from build123d import *

# Parameters (mm, degrees)
F0_W     = 112
F0_H     = 13.5
F2_DEPTH = 117.5
F3_DEPTH = 15
F4_R     = 6
F5_DEPTH = 20
F6_DEPTH = 70


with BuildPart() as f1:
    # F0 (on Front) → F1 (revolve)
    with BuildSketch(Plane.XZ):
        with BuildLine():
            Line((84.7845596923, 37.8570006367), (84.7845596923, 55.8570006367))
            Line((84.7845596923, 55.8570006367), (84.7845596923, 61.6070006367))
            Line((84.7845596923, 61.6070006367), (68.7845596923, 61.6070006367))
            ThreePointArc((68.7845596923, 61.6070006367), (66.0366424473, 58.8617238614), (62.2845596923, 57.8570006367))
            Line((62.2845596923, 57.8570006367), (-42.2154403077, 57.8570006367))
            Line((-42.2154403077, 57.8570006367), (-42.2154403077, 55.8570006367))
            Line((-42.2154403077, 55.8570006367), (-52.2154403077, 55.8570006367))
            Line((-52.2154403077, 55.8570006367), (-52.2154403077, 56.2570006367))
            Line((-52.2154403077, 56.2570006367), (-55.2154403077, 56.2570006367))
            Line((-55.2154403077, 56.2570006367), (-55.2154403077, 51.3570006367))
            Line((-55.2154403077, 51.3570006367), (-43.2154403077, 51.3570006367))
            Line((-43.2154403077, 51.3570006367), (68.7845596923, 51.3570006367))
            Line((68.7845596923, 51.3570006367), (68.7845596923, 37.8570006367))
            Line((68.7845596923, 37.8570006367), (84.7845596923, 37.8570006367))
        make_face()
        with Locations((12.7845596923, 44.6070006367)):
            Rectangle(F0_W, F0_H)
    revolve(axis=Axis((14.7845596923, 0, 37.8570006367), (1, 0, 0)))

    # F2 (cut): a face of the model
    f2_faces = [f1.faces().sort_by_distance(p)[0] for p in [
        (-43.2154403077, 0, 37.8570006367),
    ]]
    extrude(f2_faces, amount=-F2_DEPTH, mode=Mode.SUBTRACT)

    # F0 (on Front) → F3 (join, symmetric)
    with BuildSketch(Plane.XZ):
        with BuildLine():
            Line((84.7845596923, 28.8570006367), (109.7845596923, 28.8570006367))
            ThreePointArc((109.7845596923, 28.8570006367), (100.8051004109, 37.2492909907), (108.5719143545, 46.7749315225))
            ThreePointArc((108.5719143545, 46.7749315225), (96.2900045696, 50.299124768), (84.7845596923, 55.8570006367))
            Line((84.7845596923, 55.8570006367), (84.7845596923, 37.8570006367))
            Line((84.7845596923, 37.8570006367), (84.7845596923, 28.8570006367))
        make_face()
        with BuildLine():
            ThreePointArc((108.5719143545, 46.7749315225), (100.8051004109, 37.2492909907), (109.7845596923, 28.8570006367))
            ThreePointArc((109.7845596923, 28.8570006367), (116.148520723, 31.493039606), (118.7845596923, 37.8570006367))
            ThreePointArc((118.7845596923, 37.8570006367), (115.70428063, 44.6361527975), (108.5719143545, 46.7749315225))
        make_face()
    extrude(amount=F3_DEPTH, both=True)

    # F4 (on face) → F5 (join)
    with BuildSketch(Plane.XZ.offset(15)):
        with Locations((109.7845596923, 37.8570006367)):
            Circle(F4_R)
    extrude(amount=F5_DEPTH)

    # F6 (add): a face of the model
    f6_faces = [f1.faces().sort_by_distance(p)[0] for p in [
        (109.7845596923, -35, 37.8570006367),
    ]]
    extrude(f6_faces, amount=-F6_DEPTH)


solid = f1.part
Read the model definition and answer for the solid it produces. Units are mm, in the model's axes. A direction names the side the tool comes from. Round coordinates to 2 decimals unless told otherwise and drop trailing zeros. Order: outer loops, then holes, each group sorted by start corner. A loop starts at its lowest first (then second) coordinate and runs counter-clockwise, first axis right, second up.
1) The mould has two halves that part along X. Classify faces 5 (the face through (103.79, 24.86, 38.12)), 6 (the face through (-55.215, -10, 28)), 7 (the face through (-53.736, -0.809, 19.475)): released by +X, released by -X, zero draft, split by the parting line, or undercut.
2) The part is cut by section A-A on y = 0. Write down the section's boundary in (x, z), plus the area to 3 significant figures.
3) The part is cut by section C-C on y = 27.5. Write down the section's boundary in (x, z).
4) Straight lines are drawn through the part: L1, parallel to Z at x = 33, y = 0; L2, parallel to Z at x = -48.75, y = 0; L3, parallel to Y at x = -38, z = 33.5. For each, find the intervals that lie inside material, in ascending order.
5) Flat-ended cylindrical pins translate along their axes: pin 1 (1.5 mm diameter, centred on x = -33.5, z = 22, fed in from -Y); pin 2 (4 mm diameter, centred on x = 4, y = 15, fed in from +Z); pin 3 (3 mm diameter, centred on x = 61.5, z = 53, fed in from +Y). Find the tip coordinate at first contact, or state that the pin passes through.
6) The part is cut by section B-B on x = -7. Write down the section's boundary in (y, z), plus the area to 3 significant figures.
7) For faces 1 (the face through (103.79, -24.86, 38.12)), 2 (the face through (97, 0, 28.857)), 3 (the face through (-42.215, -8, 21)), 4 (the face through (74.285, 0, 38)), determine the directions among +Z, -Z, +X, -X, +Y, -Y from which every point of the face is accessible in a straight line to the end or side of a thin tool.
Resolved:
1. face 5: undercut
1. face 6: released by -X
1. face 7: zero draft
2. outline: (-55.22, 19.46) - (-52.22, 19.46) - (-52.22, 19.86) - (-42.22, 19.86) - (-42.22, 17.86) - (62.28, 17.86) arc R7.51 cw to (68.78, 14.11) - (84.78, 14.11) - (84.78, 28.86) - (109.78, 28.86) arc R9 ccw (long way) to (108.57, 46.77) arc R75 cw to (84.78, 55.86) - (84.78, 61.61) - (68.78, 61.61) arc R7.51 cw to (62.28, 57.86) - (-42.22, 57.86) - (-42.22, 55.86) - (-52.22, 55.86) - (-52.22, 56.26) - (-55.22, 56.26) - (-55.22, 51.36) - (74.28, 51.36) - (74.28, 24.36) - (-55.22, 24.36) - close
2. area: 2,850 mm2
3. outline: circle Ø12 at (109.78, 37.86)
4. L1: z = 17.86 to 24.36, 51.36 to 57.86
4. L2: z = 19.86 to 24.36, 51.36 to 55.86
4. L3: y = -19.52 to -12.78, 12.78 to 19.52
5. pin 1: stops at y = -13.11
5. pin 2: stops at z = 53.06
5. pin 3: stops at y = 14.62
6. outline: circle Ø40 at (0, 37.86); hole circle Ø27 at (0, 37.86)
6. area: 684 mm2
7. face 1: -Y
7. face 2: -Z, +X, +Y, -Y
7. face 3: none
7. face 4: -X
